```python
from build123d import *

# Parameters (mm, degrees)
CROQUIS1_R              = 1.6
SALIENTE_EXTRUIR1_DEPTH = 3
CROQUIS2_W              = 8.8
CROQUIS2_H              = 12
CROQUIS2_W_2            = 6.2
CROQUIS2_H_2            = 8.9
CROQUIS2_W_3            = 1.8
CROQUIS2_W_4            = 19
CROQUIS2_H_3            = 2
SALIENTE_EXTRUIR2_DEPTH = 5


with BuildPart() as part:
    # Croquis1 → Saliente-Extruir1 (new body)
    with BuildSketch(Plane.XY):
        Polygon((-33.05, 26.65), (-33.05, -26.65), (33.05, -26.65), (33.05, -24.15), (35.55, -21.65), (35.55, 9.45), (33.05, 11.95), (33.05, 26.65), align=None)
        with Locations((33.05, -20.05)):
            Circle(CROQUIS1_R, mode=Mode.SUBTRACT)
        with Locations((33.05, 7.85)):
            Circle(CROQUIS1_R, mode=Mode.SUBTRACT)
        with Locations((-18.85, -24.15)):
            Circle(CROQUIS1_R, mode=Mode.SUBTRACT)
        with Locations((-17.75, 24.15)):
            Circle(CROQUIS1_R, mode=Mode.SUBTRACT)
    extrude(amount=SALIENTE_EXTRUIR1_DEPTH)

    # Croquis2 → Saliente-Extruir2 (add)
    with BuildSketch(Plane.XY.offset(3)):
        with Locations((-28.65, 11.05)):
            Rectangle(CROQUIS2_W, CROQUIS2_H)
        with Locations((-29.95, -18.9)):
            Rectangle(CROQUIS2_W_2, CROQUIS2_H_2)
        with Locations((-36.15, 11.05)):
            Rectangle(CROQUIS2_W_2, CROQUIS2_H)
        with Locations((-33.95, -18.9)):
            Rectangle(CROQUIS2_W_3, CROQUIS2_H_2)
        with Locations((22.55, 24.15)):
            Rectangle(CROQUIS2_W_4, CROQUIS2_H_3)
        with Locations((-1.45, 24.15)):
            Rectangle(CROQUIS2_W_4, CROQUIS2_H_3)
    extrude(amount=SALIENTE_EXTRUIR2_DEPTH)


solid = part.part
```
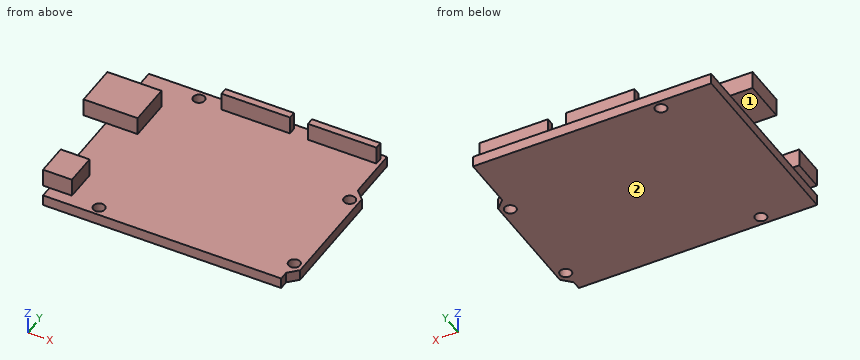
Source: CAD feature listing. Evaluate the final solid. Frame: model axes, mm. Face numbers are marked on the shaded views. A direction names the side the tool comes from. Round coordinates to 2 decimals unless told otherwise and drop trailing zeros. Loops run counter-clockwise (first coordinate to the right, second up) from the corner with the lowest first, then second, coordinate; pieces in that order, holes last. Notation, with made-up numbers: M 73.5,53.25 L 88.5,53.25 A11 cw 88.5,65.25 Z; hole C -8.75,20 d8. An arc over 180 degrees is marked long. Use a Markdown table: item, result. Add a question column.
1. Section query A-A on y = 24.15. Return the cut outline in (x, z).
2. Section query C-C on z = 1. Return the cut outline in (x, y).
3. Line query: line 1 (Y direction, x = -18.85, z = 1.4); line 2 (Z direction, x = 11, y = -1); line 3 (Y direction, x = -6.5, z = 6). Output: solid intervals per line, ascending.
4. Section query B-B on z = 6.75. Return the cut outline in (x, y), then the cut area to 3 significant figures.
5. Section query D-D on x = 25.5. Return the cut outline in (y, z).
6. Reachability of the marked faces 1 and 2 from +Z, -Z, +X, -X, +Y, -Y: full face, straight path, thin tool, end or side. Return the list, or none.
7. Contact query for flat-ended pins moving along their axis: P1, Ø1.4, axis at x = -34, y = -20, coming from the -Z side; P2, Ø2, axis at y = 24, z = 5.5, coming from the +X side; P3, Ø4, axis at x = 21.5, y = -17, coming from the +Z side. Output: stop coordinate, or through.
Reported:
| question | item | result |
|---|---|---|
| 1 | outline | M -33.05,0 L -19.35,0 L -19.35,3 L -33.05,3 Z; M -16.15,0 L 33.05,0 L 33.05,3 L 32.05,3 L 32.05,8 L 13.05,8 L 13.05,3 L 8.05,3 L 8.05,8 L -10.95,8 L -10.95,3 L -16.15,3 Z |
| 2 | outline | M -33.05,-26.65 L 33.05,-26.65 L 33.05,-24.15 L 35.55,-21.65 L 35.55,9.45 L 33.05,11.95 L 33.05,26.65 L -33.05,26.65 Z; hole C -18.85,-24.15 d3.2; hole C -17.75,24.15 d3.2; hole C 33.05,-20.05 d3.2; hole C 33.05,7.85 d3.2 |
| 3 | line 1 | y = -26.65 to -25.75, -22.55 to 22.99, 25.31 to 26.65 |
| 3 | line 2 | z = 0 to 3 |
| 3 | line 3 | y = 23.15 to 25.15 |
| 4 | outline | M -39.25,5.05 L -24.25,5.05 L -24.25,17.05 L -39.25,17.05 Z; M -34.85,-23.35 L -26.85,-23.35 L -26.85,-14.45 L -34.85,-14.45 Z; M -10.95,23.15 L 8.05,23.15 L 8.05,25.15 L -10.95,25.15 Z; M 13.05,23.15 L 32.05,23.15 L 32.05,25.15 L 13.05,25.15 Z |
| 4 | area | 327 mm² |
| 5 | outline | M -26.65,0 L 26.65,0 L 26.65,3 L 25.15,3 L 25.15,8 L 23.15,8 L 23.15,3 L -26.65,3 Z |
| 6 | face 1 | -Z, -X, +Y, -Y |
| 6 | face 2 | -Z, +X, -X, +Y, -Y |
| 7 | P1 | stops at z = 3 |
| 7 | P2 | stops at x = 32.05 |
| 7 | P3 | stops at z = 3 |
